Geometry: final body of the model. Coordinates: model frame, mm. A direction names the side the tool comes from. Give positions to 0.01 mm unless a question says otherwise; leave off trailing zeros. Write each loop counter-clockwise with the first axis right and the second up, starting at its lowest first coordinate (ties: lowest second). Pieces come first, ordered by that corner, then holes. Notation, with made-up numbers: M 85.5,77.5 L 142.5,77.5 A16 cw 142.5,106.5 Z; hole C 33,69.5 d9. An arc over 180 degrees is marked long. Use one line per item in the form item = value. Start each with the question number.
Item 1: Section query C-C on x = 0. Return loops of the section in (y, z), then the cut area to 3 significant figures.
Item 2: Pull-direction query (Y, two-part tool) for faces 5 (the cylindrical face through (-13.41, -38.06, 55.14)), 6 (the cylindrical face through (-14.91, 55.07, 33.06)), 7 (the flat face through (0.455, 12.255, 22.815)), 8 (the cylindrical face through (11.59, -38.06, 55.14)); classes: released by +Y, released by -Y, zero draft, split by the parting line, or undercut.
Item 3: Section query D-D on z = 69. Return loops of the section in (x, y), then the cut area to 4 significant figures.
Item 4: Section query A-A on y = -21. Return loops of the section in (x, z), then the cut area to 3 significant figures.
Item 5: Material intervals for line 1 along Y through (x, z) = (-12, 52); line 2 along Z through (x, y) = (14, 56.75); line 3 along X through (y, z) = (56, 40), sorted ascending. Write a range as from..to.
Item 6: Section query B-B on x = 14. Return loops of the section in (y, z).
Item 7: Contact query for flat-ended pins moving along their axis: P1, Ø8, axis at x = -8.5, y = 21.5, coming from the -Z side; P2, Ø16, axis at x = 12.5, y = -21, coming from the +Z side; P3, Ø7, axis at x = 15, z = 42, coming from the +Y side. Output: stop coordinate, or through.
Item 8: Access query for faces 1 (the flat face through (0, 28, 80)), 2 (the flat face through (0, -33, 45)), 3 (the flat face through (0, -5, 73)), 4 (the flat face through (-14, 50, 16)). Directions: +Z, -Z, +X, -X, +Y, -Y. A direction counts if a zero-diameter tool reaches every point of the face in a straight line with its end or side. Return the directions, or none.
from build123d import *

# Parameters (mm, degrees)
CROQUIS1_W              = 65
CROQUIS1_H              = 120
SALIENTE_EXTRUIR1_DEPTH = 80
CROQUIS2_W              = 15
CROQUIS2_H              = 55
CORTAR_EXTRUIR1_DEPTH   = 80
CROQUIS3_R              = 7
CORTAR_EXTRUIR2_DEPTH   = 20
CROQUIS4_R              = 7
CORTAR_EXTRUIR3_DEPTH   = 10


with BuildPart() as part:
    # Croquis1 → Saliente-Extruir1 (new body)
    with BuildSketch(Plane.XY):
        Rectangle(CROQUIS1_W, CROQUIS1_H)
    extrude(amount=SALIENTE_EXTRUIR1_DEPTH)

    # Croquis2 → Cortar-Extruir1 (cut)
    with BuildSketch(Plane(origin=(32.5, 0, 0), x_dir=(0, 0, -1), z_dir=(1, 0, 0))):
        with Locations((-72.5, -32.5)):
            Rectangle(CROQUIS2_W, CROQUIS2_H)
        Polygon((-45, -60), (-45, -5), (0, 30), (0, -60), align=None)
    extrude(amount=-CORTAR_EXTRUIR1_DEPTH, mode=Mode.SUBTRACT)

    # Croquis3 → Cortar-Extruir2 (cut)
    with BuildSketch(Plane.XY.offset(65)):
        with Locations((-12.5, -21)):
            Circle(CROQUIS3_R)
        with Locations((-12.5, -45)):
            Circle(CROQUIS3_R)
        with Locations((12.5, -21)):
            Circle(CROQUIS3_R)
        with Locations((12.5, -45)):
            Circle(CROQUIS3_R)
    extrude(amount=-CORTAR_EXTRUIR2_DEPTH, mode=Mode.SUBTRACT)

    # Croquis4 → Cortar-Extruir3 (cut)
    with BuildSketch(Plane(origin=(0, 60, 0), x_dir=(1, 0, 0), z_dir=(0, 1, 0))):
        with Locations((14, -16)):
            Circle(CROQUIS4_R)
        with Locations((-14, -16)):
            Circle(CROQUIS4_R)
        with Locations((14, -40)):
            Circle(CROQUIS4_R)
        with Locations((-14, -40)):
            Circle(CROQUIS4_R)
    extrude(amount=-CORTAR_EXTRUIR3_DEPTH, mode=Mode.SUBTRACT)


solid = part.part
Answer sheet:
q1.outline = M -60,45 L -5,45 L 30,0 L 60,0 L 60,80 L -5,80 L -5,65 L -60,65 Z
q1.area = 5,510 mm2
q2.face_5 = undercut
q2.face_6 = zero draft
q2.face_7 = released by -Y
q2.face_8 = undercut
q3.outline = M -32.5,-5 L 32.5,-5 L 32.5,60 L -32.5,60 Z
q3.area = 4,225 mm2
q4.outline = M -32.5,45 L -19.5,45 L -19.5,65 L -32.5,65 Z; M -5.5,45 L 5.5,45 L 5.5,65 L -5.5,65 Z; M 19.5,45 L 32.5,45 L 32.5,65 L 19.5,65 Z
q4.area = 740 mm2
q5.line_1 = -60..-51.98, -38.02..-27.98, -14.02..60
q5.line_2 = 0..9, 23..33, 47..80
q5.line_3 = -32.5..-21, -7..7, 21..32.5
q6.outline = M -60,45 L -51.84,45 L -51.84,65 L -60,65 Z; M -38.16,45 L -27.84,45 L -27.84,65 L -38.16,65 Z; M -14.16,45 L -5,45 L 30,0 L 60,0 L 60,9 L 50,9 L 50,23 L 60,23 L 60,33 L 50,33 L 50,47 L 60,47 L 60,80 L -5,80 L -5,65 L -14.16,65 Z
q7.P1 = 5.79
q7.P2 = 65
q7.P3 = 50
q8.face_1 = +Z, +X, -X, +Y, -Y
q8.face_2 = -Z, +X, -X, -Y
q8.face_3 = +Z, +X, -X, -Y
q8.face_4 = +Y
